Here's how the part is built. I have some questions about the finished solid (model axes, mm). A direction names the side the tool comes from. Round coordinates to 2 decimals unless told otherwise and drop trailing zeros. Loops run counter-clockwise (first coordinate to the right, second up) from the corner with the lowest first, then second, coordinate; pieces in that order, holes last. Notation, with made-up numbers: M 12,-21.75 L 71,-21.75 A19 ccw 71,12.25 Z; hole C -12.75,52.5 d7. An arc over 180 degrees is marked long. Write item = value, one per line. Start each with the question number.
Autodesk Inventor part; units mm, degrees
ref_plane "YZ Plane" through (0, 0, 0) normal (1, 0, 0) x (0, 1, 0)
ref_plane "XZ Plane" through (0, 0, 0) normal (0, 1, 0) x (-1, 0, 0)
ref_plane "XY Plane" through (0, 0, 0) normal (0, 0, 1) x (1, 0, 0)
sketch "Sketch1" plane through (0, 0, 0) normal (0, 1, 0) x (-1, 0, 0)
  line L0 (0, 0) -> (80, 0)
  line L1 (20, 5) -> (0, 5)
  line L2 (0, 5) -> (0, 0)
  line L3 (46.5184, 5) -> (46.5184, 80)
  circle A0 centre (26.5184, 80) radius 20
  line L4 (26.5184, 100) -> (-123.4816, 100)
  circle A1 centre (-123.4816, 80) radius 20
  line L5 (-123.4816, 60) -> (-39.7913, 60)
  arc A2 (20, 5) -> (-39.7913, 60) centre (-39.7913, 0) ccw
  line L6 (46.5184, 5) -> (66.5184, 5)
  line L7 (66.5184, 5) -> (66.5184, 0)
  line L8 (66.5184, 0) -> (46.5184, 0)
  point P0 (16.5184, 60)
  dimension "d1" = 75
  dimension "d2" = 40
  dimension "d3" = 150
  dimension "d4" = 140
  dimension "d7" = 40
  dimension "d10" = 5
  dimension "d11" = 5
extrude "Extrusion1" add sketch "Sketch1" along normal blind 15
sketch "Sketch4" plane through (0, 0, 0) normal (0, -1, 0) x (1, 0, 0)
  line L0 (-26.5184, 100) -> (123.4816, 100)
  arc A0 (-26.5184, 100) -> (-46.5184, 80) centre (-26.5184, 80) ccw
  line L1 (-46.5184, 5) -> (-46.5184, 80)
  line L2 (-66.5184, 5) -> (-46.5184, 5)
  line L3 (-66.5184, 0) -> (-66.5184, 5)
  line L4 (0, 0) -> (-66.5184, 0)
  line L5 (0, 5) -> (0, 0)
  line L6 (-20, 5) -> (0, 5)
  arc A1 (39.7913, 60) -> (-20, 5) centre (39.7913, 0) ccw
  line L7 (123.4816, 60) -> (39.7913, 60)
  arc A2 (123.4816, 60) -> (123.4816, 100) centre (123.4816, 80) ccw
  line L8 (-20, 5) -> (-46.5184, 5)
extrude "Extrusion3" add sketch "Sketch4" along normal blind 20 and the other way blind 35 contours L8 L6 L5 L4 L3 L2
sketch "Sketch5" plane through (0, 0, 0) normal (0, -1, 0) x (1, 0, 0)
  line L0 (-46.5184, 5) -> (-20, 5)
  arc A0 (39.7913, 60) -> (-20, 5) centre (39.7913, 0) ccw
  line L1 (123.4816, 60) -> (39.7913, 60)
  arc A1 (123.4816, 60) -> (123.4816, 100) centre (123.4816, 80) ccw
  line L2 (-26.5184, 100) -> (123.4816, 100)
  arc A2 (-26.5184, 100) -> (-46.5184, 80) centre (-26.5184, 80) ccw
  line L3 (-46.5184, 5) -> (-46.5184, 80)
  arc A3 (39.7913, 62.5) -> (-22.2571, 7.5) centre (39.7913, 0) ccw
  line L4 (-22.2571, 7.5) -> (-44.0184, 7.5)
  line L5 (-44.0184, 7.5) -> (-44.0184, 80)
  arc A4 (-26.5184, 97.5) -> (-44.0184, 80) centre (-26.5184, 80) ccw
  line L6 (-26.5184, 97.5) -> (123.4816, 97.5)
  arc A5 (123.4816, 62.5) -> (123.4816, 97.5) centre (123.4816, 80) ccw
  line L7 (123.4816, 62.5) -> (39.7913, 62.5)
  point P0 (0, 0)
  dimension "d29" = 2.5
extrude "Extrusion4" cut sketch "Sketch5" against normal blind 5 contours A3 L4 L5 A4 L6 A5 L7
sketch "Sketch6" plane through (0, 15, 0) normal (0, 1, 0) x (1, 0, 0)
  line L0 (-20, -5) -> (-46.5184, -5)
  line L1 (-46.5184, -5) -> (-46.5184, -80)
  arc A0 (-46.5184, -80) -> (-26.5184, -100) centre (-26.5184, -80) ccw
  line L2 (-26.5184, -100) -> (123.4816, -100)
  arc A1 (123.4816, -100) -> (123.4816, -60) centre (123.4816, -80) ccw
  line L3 (123.4816, -60) -> (39.7913, -60)
  arc A2 (-20, -5) -> (39.7913, -60) centre (39.7913, 0) ccw
  line L4 (-44.0184, -80) -> (-44.0184, -7.5)
  line L5 (-44.0184, -7.5) -> (-22.2571, -7.5)
  arc A3 (-22.2571, -7.5) -> (39.7913, -62.5) centre (39.7913, 0) ccw
  line L6 (39.7913, -62.5) -> (123.4816, -62.5)
  arc A4 (123.4816, -97.5) -> (123.4816, -62.5) centre (123.4816, -80) ccw
  line L7 (123.4816, -97.5) -> (-26.5184, -97.5)
  arc A5 (-44.0184, -80) -> (-26.5184, -97.5) centre (-26.5184, -80) ccw
  point P0 (0, 0)
  dimension "d32" = 2.5
extrude "Extrusion5" cut sketch "Sketch6" against normal blind 5 contours L4 L5 A3 L6 A4 L7 A5
sketch "Sketch7" plane through (0, 10, 0) normal (0, 1, 0) x (1, 0, 0)
  line L0 (123.4816, -97.5) -> (-26.5184, -97.5)
  line L1 (39.7913, -62.5) -> (123.4816, -62.5)
  line L2 (123.4816, -62.5) -> (39.7913, -62.5)
  line L3 (118.4816, -62.5) -> (118.4816, -80)
  circle A0 centre (118.4816, -80) radius 4
  line L4 (-44.0184, -80) -> (-44.0184, -7.5)
  circle A1 centre (88.4816, -80) radius 4
  circle A2 centre (58.4816, -80) radius 4
  circle A3 centre (28.4816, -80) radius 4
  circle A4 centre (-1.5184, -80) radius 4
  circle A5 centre (-31.5184, -80) radius 4
  arc A6 (123.4816, -97.5) -> (123.4816, -62.5) centre (123.4816, -80) ccw
  circle A7 centre (-31.5184, -50) radius 4
  point P0 (0, 0)
  dimension "d35" = 35
  dimension "d36" = 17.5
  dimension "d37" = 8
  dimension "d39" = 8
  dimension "d41" = 8
  dimension "d43" = 8
  dimension "d45" = 8
  dimension "d46" = 8
  dimension "d47" = 30
  dimension "d48" = 30
  dimension "d49" = 30
  dimension "d50" = 30
  dimension "d51" = 5
  dimension "d52" = 30
  dimension "d53" = 8
  dimension "d54" = 30
extrude "Extrusion6" cut sketch "Sketch7" against normal blind 8
sketch "Sketch8" plane through (0, 35, 0) normal (0, 0, -1) x (-1, 0, 0)
  line L0 (20, -20) -> (46.5184, -20)
  line L1 (46.5184, -35) -> (20, -35)
  line L2 (20, -35) -> (20, -20)
  line L3 (46.5184, -35) -> (46.5184, -20)
  line L4 (0, 0) -> (66.5184, 0)
  line L5 (66.5184, -55) -> (0, -55)
  circle A0 centre (10, -27.5) radius 5
  circle A1 centre (57.0363, -27.5) radius 5
  point P0 (0, -35)
  dimension "d57" = 20
  dimension "d58" = 20
  dimension "d59" = 10
  dimension "d60" = 10
  dimension "d61" = 10
extrude "Extrusion7" cut sketch "Sketch8" against normal blind 10 contours A0 | A1
equation "\"d55\" = d39"
properties part number "Pylon2"
Item 1: We'd pull the mould along X, two halves only. Please class faces 6 (the flat face through (47, 7, 100)), 7 (the flat face through (0, 7, 3)), 8 (the cylindrical face through (-2.139, 12.535, 46.347)): released by +X, released by -X, zero draft, split by the parting line, or undercut.
Item 2: I want a section at B-B, the plane x = -3. List the corners of the cut face in (y, z) for me.
Item 3: For faces 1 (the flat face through (28, 15, 60)), 2 (the flat face through (82, 7, 60)), 3 (the flat face through (27, 5, 73)), 4 (the flat face through (81, 13, 62.5)), 5 (the cylindrical face through (-14.77, 9, 2.46)), which set-ups out of +Z, -Z, +X, -X, +Y, -Y let a thin tool reach every point of the face, with its end or its side?
Item 4: Will these pins go through, and if not, where does the flat tip stop? pin 1 Ø2.5 at (y, z) = (13, 26.5) entering from +X; pin 2 Ø5.5 at (x, y) = (-37, 1.5) entering from +Z; pin 3 Ø1.5 at (x, y) = (34.5, 3.5) entering from -Z; pin 4 Ø10 at (y, z) = (-5.5, 12) entering from -X.
Item 5: I want a section at C-C, the plane z = 50. List the corners of the cut face in (x, y) for me, then the cut area to 3 significant figures.
Item 6: I want a section at D-D, the plane x = 43.5. List the corners of the cut face in (y, z) for me, then the cut area to 3 significant figures.
Item 7: Please list where these lines run through material, in increasing order: line 1 (Y direction, x = -10, z = 3.4); line 2 (Y direction, x = 23.5, z = 95.5); line 3 (Z direction, x = -40.5, y = -16). Write a range as [from, to].
Item 8: I want a section at A-A, the plane y = 7.5. State how many separate pieces and enclosed holes the cut face has, then the cut area to 3 significant figures.
Worked out:
q1.face_6 = zero draft
q1.face_7 = released by +X
q1.face_8 = undercut
q2.outline = M -20,0 L 35,0 L 35,5 L -20,5 Z; M 0,42.06 L 15,42.06 L 15,45.55 L 10,45.55 L 10,76.28 L 5,76.28 L 5,45.55 L 0,45.55 Z; M 0,97.5 L 5,97.5 L 5,83.72 L 10,83.72 L 10,97.5 L 15,97.5 L 15,100 L 0,100 Z
q3.face_1 = +Z, +X, -X, +Y
q3.face_2 = -Z, +X, +Y, -Y
q3.face_3 = -Y
q3.face_4 = +Y
q3.face_5 = -Z
q4.pin_1 = -13.41
q4.pin_2 = 98.45
q4.pin_3 = 59.7
q4.pin_4 = through
q5.outline = M -46.52,0 L -44.02,0 L -44.02,5 L -35.52,5 L -35.52,10 L -44.02,10 L -44.02,15 L -46.52,15 Z; M -27.52,5 L 2.29,5 L 2.29,0 L 6.63,0 L 6.63,15 L 2.29,15 L 2.29,10 L -27.52,10 Z
q5.area = 294 mm2
q6.outline = M 0,60 L 15,60 L 15,62.5 L 10,62.5 L 10,97.5 L 15,97.5 L 15,100 L 0,100 L 0,97.5 L 5,97.5 L 5,62.5 L 0,62.5 Z
q6.area = 250 mm2
q7.line_1 = [-20, 2.5], [12.5, 35]
q7.line_2 = [5, 10]
q7.line_3 = [0, 5]
q8.separate_pieces = 3
q8.enclosed_holes = 7
q8.area = 9,440 mm2
